Check sheet for the modelled part. Datum: model origin and axes. Units: mm. Coordinates: 2 decimals unless noted, no trailing zeros. Loops run counter-clockwise (first coordinate to the right, second up) from the corner with the lowest first, then second, coordinate; pieces in that order, holes last. Notation, with made-up numbers: M -14.75,46.25 L 21.25,46.25 A12 ccw 21.25,55.25 Z; hole C 27,31 d5. An arc over 180 degrees is marked long. Return JSON: item names as keys, results as strings.
from build123d import *

# Parameters (mm, degrees)
BOSS_EXTRUDE1_DEPTH = 40
SKETCH4_R           = 15


with BuildPart() as part:
    # Sketch1 → Boss-Extrude1 (new body)
    with BuildSketch(Plane.XY):
        Polygon((150, 50), (0, 0), (150, 0), align=None)
    extrude(amount=BOSS_EXTRUDE1_DEPTH)

    # Cut-Sweep1: sweep along a curve in space
    with BuildLine() as cut_sweep1_path:
        Line((150, 50, 20), (0, 0, 20))
    # Sketch4 → Cut-Sweep1 (sweep, cut)
    with BuildSketch(Plane(origin=(150, 50, 0), x_dir=(0, 0, 1), z_dir=(-0.948683298, -0.316227766, 0))):
        with Locations((20, 0)):
            Circle(SKETCH4_R)
    sweep(path=cut_sweep1_path.line, mode=Mode.SUBTRACT)


solid = part.part
1) Section check B-B on z = 19.5. Record the cut outline in (x, y).
Answers:
{"outline": "M 47.41,0 L 150,0 L 150,34.2 Z"}
2) Draft check along Z on faces 1 (the face through (95.36, 15.98, 19.67)), 2 (the face through (91, 0, 20)), 3 (the face through (107, 14, 40)). Enter one of: +Z half, -Z half, draft (parallel to the pull), parting line (faces both ways), or undercut.
Answers:
{"face 1": "undercut", "face 2": "draft", "face 3": "+Z half"}
3) Scan lines: line 1 along Z through (x, y) = (113, 36); line 2 along Z through (x, y) = (87, 19); line 3 along Y through (x, z) = (139.5, 29). Record each from-to range of solid material in increasing order. Write a range as [from, to].
Answers:
{"line 1": "[0, 5.08], [34.92, 40]", "line 2": "[0, 8.38], [31.62, 40]", "line 3": "[0, 33.85]"}
4) Section check A-A on z = 37.5. Record the cut outline in (x, y).
Answers:
{"outline": "M 0,0 L 150,0 L 150,50 Z"}
5) Go/stop test with flat-tipped pins: pin 1 Ø2 at (x, z) = (96, 20) entering from +Y; pin 2 Ø1 at (y, z) = (44.5, 31.5) entering from +X; pin 3 Ø2 at (x, z) = (35.5, 7.5) entering from +Y; pin 4 Ø5 at (x, z) = (104.5, 6) entering from +Y. Record where each tip stops, or that it passes through.
Answers:
{"pin 1": "y = 16.52", "pin 2": "through", "pin 3": "y = 4.97", "pin 4": "y = 35.6"}
